Geometry: final body of the model. Coordinates: model frame, mm. A direction names the side the tool comes from. Give positions to 0.01 mm unless a question says otherwise; leave off trailing zeros. Write each loop counter-clockwise with the first axis right and the second up, starting at its lowest first coordinate (ties: lowest second). Pieces come first, ordered by that corner, then holes.
Q1. Pin query (flat end, axial travel): pin 1 (8 mm diameter, centred on y = -180, z = -791, fed in from -X); pin 2 (2 mm diameter, centred on y = 173, z = -1483, fed in from -X); pin 3 (4 mm diameter, centred on y = 189, z = -889, fed in from +X). Return the tip coordinate at first contact, or that it passes through.
Q2. Line query: L1, parallel to Y at x = -1896.5, z = -411; L2, parallel to Z at x = -712.5, y = -83; L3, parallel to Z at x = -355.5, y = -151. Output: solid intervals per line, ascending.
Q3. Cut plane D-D on z = -1827.5. Return the cut outline in (x, y).
Q4. Draft query along Y for faces 1 (the face through (-937, -248, -965)), 2 (the face through (-699.29, -3.5, -714.84)), 3 (the face through (-950, -250, -978)). Return one class per face: pulls with the +Y half, pulls with the -Y half, needs draft (parallel to the pull), parting line crosses it, or undercut.
Q5. Cut plane A-A on y = -199.5. Return the cut outline in (x, z).
Q6. Cut plane B-B on z = -387. Return the cut outline in (x, y).
Q7. Reachability of faces 4 (the face through (-1398.578, 3.5, -1429.678)), 5 (the face through (-1397.18, -3.47, -1428.25)) from +Z, -Z, +X, -X, +Y, -Y: full face, straight path, thin tool, end or side. Return the list, or none.
Q8. Cut plane C-C on x = -127.5. Return the cut outline in (y, z) (3 decimals).
```python
from build123d import *

# Parameters (mm, degrees)
SKETCH1_W   = 1000
SKETCH1_H   = 500
SKETCH1_W_2 = 996
SKETCH1_H_2 = 496


with BuildPart() as part:
    # Sweep-Thin1: sweep along a path in ElbowArc
    with BuildLine(Plane(origin=(0, 0, 0), x_dir=(1, 0, 0), z_dir=(0, 1, 0))) as sweep_thin1_path:
        ThreePointArc((0, 1500), (-1060.66017178, 1060.66017178), (-1500, 0))
    # Sketch1 → Sweep-Thin1 (sweep)
    with BuildSketch(Plane(origin=(0, 0, 0), x_dir=(0, 0, -1), z_dir=(1, 0, 0))):
        with Locations((1500, 0)):
            Rectangle(SKETCH1_W, SKETCH1_H)
        with Locations((1500, 0)):
            Rectangle(SKETCH1_W_2, SKETCH1_H_2, mode=Mode.SUBTRACT)
    sweep(path=sweep_thin1_path.line)


solid = part.part
```
Data:
1. pin 1: stops at x = -1838.65
1. pin 2: stops at x = -1343.01
1. pin 3: stops at x = -454
2. L1: y = -250 to -248, 248 to 250
2. L2: z = -1868.78 to -1866.64, -704.52 to -701.67
2. L3: z = -1968.15 to -1966.12, -936.82 to -934.68
3. outline: (-812.55, -250) - (0, -250) - (0, -248) - (-807.62, -248) - (-807.62, 248) - (0, 248) - (0, 250) - (-812.55, 250) - close
4. face 1: undercut
4. face 2: needs draft
4. face 3: pulls with the -Y half
5. outline: (-2000, 0) arc R2000 ccw to (0, -2000) - (0, -1998) arc R1998 cw to (-1998, 0) - close; (-1002, 0) arc R1002 ccw to (0, -1002) - (0, -1000) arc R1000 cw to (-1000, 0) - close
6. outline: (-1962.2, -250) - (-922.08, -250) - (-922.08, 250) - (-1962.2, 250) - close; hole (-1960.16, -248) - (-924.25, -248) - (-924.25, 248) - (-1960.16, 248) - close
7. face 4: -Z, -X, +Y, -Y
7. face 5: none
8. outline: (-250, -1995.932) - (250, -1995.932) - (250, -991.839) - (-250, -991.839) - close; hole (-248, -1993.928) - (248, -1993.928) - (248, -993.855) - (-248, -993.855) - close
